```python
from build123d import *

# Parameters (mm, degrees)
F0_R     = 2.05
F1_DEPTH = 8
F2_R     = 3.55
F2_R_2   = 2.05
F3_DEPTH = 1
F4_R     = 0.5


with BuildPart() as f1:
    # F0 (on Top) → F1 (new body)
    with BuildSketch(Plane.XY):
        Circle(F0_R)
    extrude(amount=F1_DEPTH)

    # F2 (on face) → F3 (join)
    with BuildSketch(Plane(origin=(0, 0, 0), x_dir=(1, 0, 0), z_dir=(0, 0, -1))):
        Circle(F2_R)
        Circle(F2_R_2, mode=Mode.SUBTRACT)
        Circle(F2_R_2)
    extrude(amount=F3_DEPTH)

    # F4
    f4_edges = [f1.edges().sort_by_distance(p)[0] for p in [
        (-3.55, 0, -1),
    ]]
    fillet(f4_edges, radius=F4_R)


solid = f1.part
```
Geometry check sheet. Reference: the model listing, model coordinates, mm. A direction names the side the tool comes from. Round coordinates to 2 decimals unless told otherwise and drop trailing zeros. Order: outer loops, then holes, each group sorted by start corner. A loop starts at its lowest first (then second) coordinate and runs counter-clockwise, first axis right, second up. Notation, with made-up numbers: M -9.75,81.5 L 47.25,81.5 A26 ccw 47.25,118.5 Z; hole C -34.5,-14.75 d6. An arc over 180 degrees is marked long. Write item = value, one per line.
Q1. Set-up check for faces 1 (the flat face through (0, 0, 8)), 2 (the cylindrical face through (-0.267, 2.033, 3.944)): record each of +Z, -Z, +X, -X, +Y, -Y from which the full face is reachable in a straight line by a thin tool's end or side.
Answer block:
face_1 = +Z, +X, -X, +Y, -Y
face_2 = +Z
Q2. Depth check by flat-ended pin: pin 1 Ø3 at (x, z) = (-1.5, 4.5) entering from +Y; pin 2 Ø1.5 at (x, z) = (-1, 1.5) entering from -Y; pin 3 Ø1 at (y, z) = (-1, 4) entering from +X. Enter the tip coordinate at first touch or a pass-through.
Answer block:
pin_1 = 2.05
pin_2 = -2.03
pin_3 = 1.99
Q3. Release check for a two-part mould opening along X. For faces 3 (the cylindrical face through (-0.46, -3.52, -0.25)), 4 (the flat face through (0, 0, -1)) record: released by +X, released by -X, zero draft, split by the parting line, or undercut.
Answer block:
face_3 = split by the parting line
face_4 = zero draft
Q4. Scan lines: line 1 (Z direction, x = 2, y = 0.75); line 2 (Y direction, x = 1, z = 5.75); line 3 (Y direction, x = 1.5, z = 3.5). Record each from-to range of solid material in increasing order.
Answer block:
line_1 = -1 to 0
line_2 = -1.79 to 1.79
line_3 = -1.4 to 1.4
Q5. Section check C-C (z = 3). Enter the section's corners in (x, y), plus the area to 3 significant figures.
Answer block:
outline = C 0,0 d4.1
area = 13.2 mm^2
Q6. Section check A-A (x = 0). Enter the section's corners in (y, z).
Answer block:
outline = M -3.55,-0.5 A0.5 ccw -3.05,-1 L 3.05,-1 A0.5 ccw 3.55,-0.5 L 3.55,0 L 2.05,0 L 2.05,8 L -2.05,8 L -2.05,0 L -3.55,0 Z
